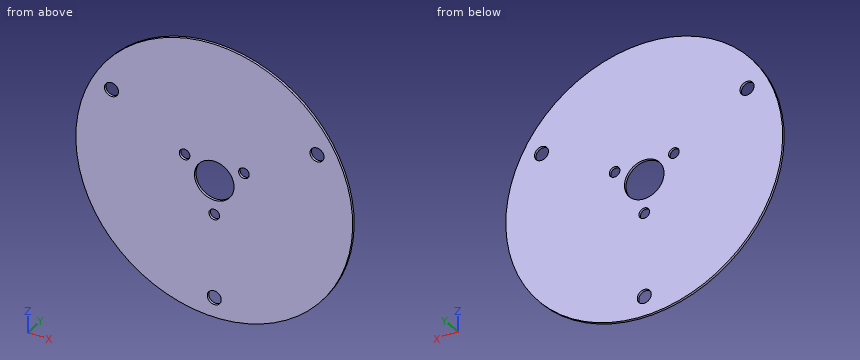
```python
from build123d import *

# Parameters (mm, degrees)
SKETCH1_R            = 44.45
BOSS_EXTRUDE1_DEPTH  = 0.8
M4_CLEARANCE_HOLE1_D = 4.5
SKETCH11_R           = 6.35
CUT_EXTRUDE1_DEPTH   = 63.866883174
M3_CLEARANCE_HOLE1_D = 3.4


with BuildPart() as part:
    # Sketch1 → Boss-Extrude1 (new body)
    with BuildSketch(Plane(origin=(0, 0, 0), x_dir=(1, 0, 0), z_dir=(0, 1, 0))):
        with Locations(Location((0, 0, 0), (0, 0, 270))):
            Circle(SKETCH1_R)
    extrude(amount=BOSS_EXTRUDE1_DEPTH)

    # M4 Clearance Hole1 (through all)
    with Locations(Plane(origin=(0, 0.8, 0), x_dir=(1, 0, 0), z_dir=(0, 1, 0))):
        with Locations((0, 38.1), (-32.995567884, -19.05), (32.995567884, -19.05)):
            Hole(M4_CLEARANCE_HOLE1_D / 2)

    # Sketch11 → Cut-Extrude1 (cut, through all)
    with BuildSketch(Plane(origin=(0, 0.8, 0), x_dir=(1, 0, 0), z_dir=(0, 1, 0))):
        with Locations(Location((0, 0, 0), (0, 0, 270))):
            Circle(SKETCH11_R)
    extrude(amount=-CUT_EXTRUDE1_DEPTH, mode=Mode.SUBTRACT)

    # M3 Clearance Hole1 (through all)
    with Locations(Plane(origin=(0, 0.8, 0), x_dir=(1, 0, 0), z_dir=(0, 1, 0))):
        with Locations((0, 11), (-9.526279442, -5.5), (9.526279442, -5.5)):
            Hole(M3_CLEARANCE_HOLE1_D / 2)


solid = part.part
```
Part model, mm, in its own coordinate system. Coordinates: 2 decimals unless noted, no trailing zeros. Order: outer loops, then holes, each group sorted by start corner. A loop starts at its lowest first (then second) coordinate and runs counter-clockwise, first axis right, second up. Notation, with made-up numbers: (56, 9) - (91, 9) arc R11 cw to (91, 14) - close; hole circle Ø3 at (49.5, -21). An arc over 180 degrees is marked (long way). Return JSON: item names as keys, results as strings. Group by question number.
Item 1: Cut at B-B (y = 0.4). List the corners of the cut face in (x, z), plus the area to 3 significant figures.
Item 2: Cut at A-A (x = 0). List the corners of the cut face in (y, z).
Item 3: Cut at D-D (z = 19.05). List the corners of the cut face in (x, y), plus the area to 3 significant figures.
Item 4: Drill centre lines: probe 1 along Z at (x, y) = (0.5, 0.3); probe 2 along X at (y, z) = (0.5, 5.5); probe 3 along X at (y, z) = (0.65, 19.05). Where is each one in solid material? Low to high. Write a range as from..to.
Item 5: Cut at C-C (z = -38.1). List the corners of the cut face in (x, y), plus the area to 3 significant figures.
Check values:
{
 "1": {"outline": "circle Ø88.9 at (0, 0); hole circle Ø4.5 at (-33, 19.05); hole circle Ø3.4 at (-9.53, 5.5); hole circle Ø12.7 at (0, 0); hole circle Ø4.5 at (0, -38.1); hole circle Ø3.4 at (0, -11); hole circle Ø3.4 at (9.53, 5.5); hole circle Ø4.5 at (33, 19.05)", "area": "6,010 mm2"},
 "2": {"outline": "(0, -44.45) - (0.8, -44.45) - (0.8, -40.35) - (0, -40.35) - close; (0, -35.85) - (0.8, -35.85) - (0.8, -12.7) - (0, -12.7) - close; (0, -9.3) - (0.8, -9.3) - (0.8, -6.35) - (0, -6.35) - close; (0, 6.35) - (0.8, 6.35) - (0.8, 44.45) - (0, 44.45) - close"},
 "3": {"outline": "(-40.16, 0) - (-35.25, 0) - (-35.25, 0.8) - (-40.16, 0.8) - close; (-30.75, 0) - (30.75, 0) - (30.75, 0.8) - (-30.75, 0.8) - close; (35.25, 0) - (40.16, 0) - (40.16, 0.8) - (35.25, 0.8) - close", "area": "57.1 mm2"},
 "4": {"probe 1": "z = -44.45..-40.29, -35.91..-12.62, -9.38..-6.33, 6.33..44.45", "probe 2": "x = -44.11..-11.23, -7.83..-3.17, 3.17..7.83, 11.23..44.11", "probe 3": "x = -40.16..-35.25, -30.75..30.75, 35.25..40.16"},
 "5": {"outline": "(-22.9, 0) - (-2.25, 0) - (-2.25, 0.8) - (-22.9, 0.8) - close; (2.25, 0) - (22.9, 0) - (22.9, 0.8) - (2.25, 0.8) - close", "area": "33.0 mm2"}
}
